```python
from build123d import *

# Parameters (mm, degrees)
F2_R = 0.762
F3_R = 0.254


with BuildPart() as f1:
    # F0 (on Right) → F1 (revolve)
    with BuildSketch(Plane.YZ):
        Polygon((-20.32, 0), (25.4, 0), (25.4, 12.7), (0, 12.7), (0, 4.572), (-20.32, 4.043167), align=None)
    revolve(axis=Axis((0, 2.54, 0), (0, 1, 0)))

    # F2
    f2_edges = [f1.edges().sort_by_distance(p)[0] for p in [
        (0, 0, -4.572),
    ]]
    fillet(f2_edges, radius=F2_R)

    # F3
    f3_edges = [f1.edges().sort_by_distance(p)[0] for p in [
        (0, 0, -12.7),
        (0, 25.4, -12.7),
        (0, -20.32, -4.043167),
    ]]
    fillet(f3_edges, radius=F3_R)


solid = f1.part
```
Check sheet for the modelled part. Datum: model origin and axes. Units: mm. A direction names the side the tool comes from. Give positions to 0.01 mm unless a question says otherwise; leave off trailing zeros. Write each loop counter-clockwise with the first axis right and the second up, starting at its lowest first coordinate (ties: lowest second). Pieces come first, ordered by that corner, then holes. Notation, with made-up numbers: (49, -22) - (82, -22) arc R19 cw to (82, -13) - close; hole circle Ø6 at (-3.5, -4). An arc over 180 degrees is marked (long way). Answer as a JSON object with one key per item and string values. Group by question number.
1) Depth check by flat-ended pin: P1, Ø1.5, axis at y = -2.5, z = -9.5, coming from the +X side; P2, Ø1.5, axis at y = -15.5, z = 2.5, coming from the +X side; P3, Ø2, axis at x = -4.5, y = -6, coming from the -Z side; P4, Ø8, axis at x = 3.5, y = -2.5, coming from the -Z side. Enter the tip coordinate at first touch or a pass-through.
2) Thickness scan on probe 1 along Y at (x, z) = (-10.75, 6); probe 2 along X at (y, z) = (19, 2.5); probe 3 along X at (y, z) = (15, 0.5). Record the ranges inside material, lowest first. Write a range as from..to.
3) Sectioned sample at C-C (y = 13.5). Record the cut outline in (x, z).
4) Sectioned sample at B-B (z = 0). Record the cut outline in (x, y).
5) Release check for a two-part mould opening along Z. For faces 1 (the face through (0, -20.32, 0)), 2 (the face through (1.29, -10.54, 4.1)) record: pulls with the +Z half, pulls with the -Z half, needs draft (parallel to the pull), parting line crosses it, or undercut.
6) Access from +Z, -Z, +X, -X, +Y, -Y to the whole of each face (thin tool, end or side, straight path). Record for faces 3 (the face through (-5, 0, 3)), 4 (the face through (-12.4, 12.53, -2.75)).
7) Sectioned sample at A-A (x = 0). Record the cut outline in (y, z).
8) Sectioned sample at D-D (y = -3). Record the cut outline in (x, z).
Geometry results:
{
 "1": {"P1": "passes through", "P2": "stops at x = 3.78", "P3": "stops at z = -2.69", "P4": "stops at z = -12.69"},
 "2": {"probe 1": "y = 0..25.4", "probe 2": "x = -12.45..12.45", "probe 3": "x = -12.69..12.69"},
 "3": {"outline": "circle Ø25.4 at (0, 0)"},
 "4": {"outline": "(-12.7, 0.25) arc R0.25 ccw to (-12.45, 0) - (-5.31, 0) arc R0.76 cw to (-4.55, -0.74) - (-4.05, -20.07) arc R0.25 ccw to (-3.8, -20.32) - (3.8, -20.32) arc R0.25 ccw to (4.05, -20.07) - (4.55, -0.74) arc R0.76 cw to (5.31, 0) - (12.45, 0) arc R0.25 ccw to (12.7, 0.25) - (12.7, 25.15) arc R0.25 ccw to (12.45, 25.4) - (-12.45, 25.4) arc R0.25 ccw to (-12.7, 25.15) - close"},
 "5": {"face 1": "needs draft", "face 2": "parting line crosses it"},
 "6": {"face 3": "-Y", "face 4": "+Y, -Y"},
 "7": {"outline": "(-20.32, -3.8) arc R0.25 ccw to (-20.07, -4.05) - (-0.74, -4.55) arc R0.76 cw to (0, -5.31) - (0, -12.45) arc R0.25 ccw to (0.25, -12.7) - (25.15, -12.7) arc R0.25 ccw to (25.4, -12.45) - (25.4, 12.45) arc R0.25 ccw to (25.15, 12.7) - (0.25, 12.7) arc R0.25 ccw to (0, 12.45) - (0, 5.31) arc R0.76 cw to (-0.74, 4.55) - (-20.07, 4.05) arc R0.25 ccw to (-20.32, 3.8) - close"},
 "8": {"outline": "circle Ø8.99 at (0, 0)"}
}
